Input: dimensioned drawing with shaded views. Units: mm. Origin: part minimum x, y, z. Coordinates: 2 decimals unless noted, no trailing zeros. Write each loop counter-clockwise with the first axis right and the second up, starting at its lowest first coordinate (ties: lowest second). Pieces come first, ordered by that corner, then holes. Notation, with made-up numbers: M 31.25,-34 L 76.25,-34 A16 ccw 76.25,-10 Z; hole C 22,8 d4. An arc over 180 degrees is marked long. Use one line per item in the form item = value.
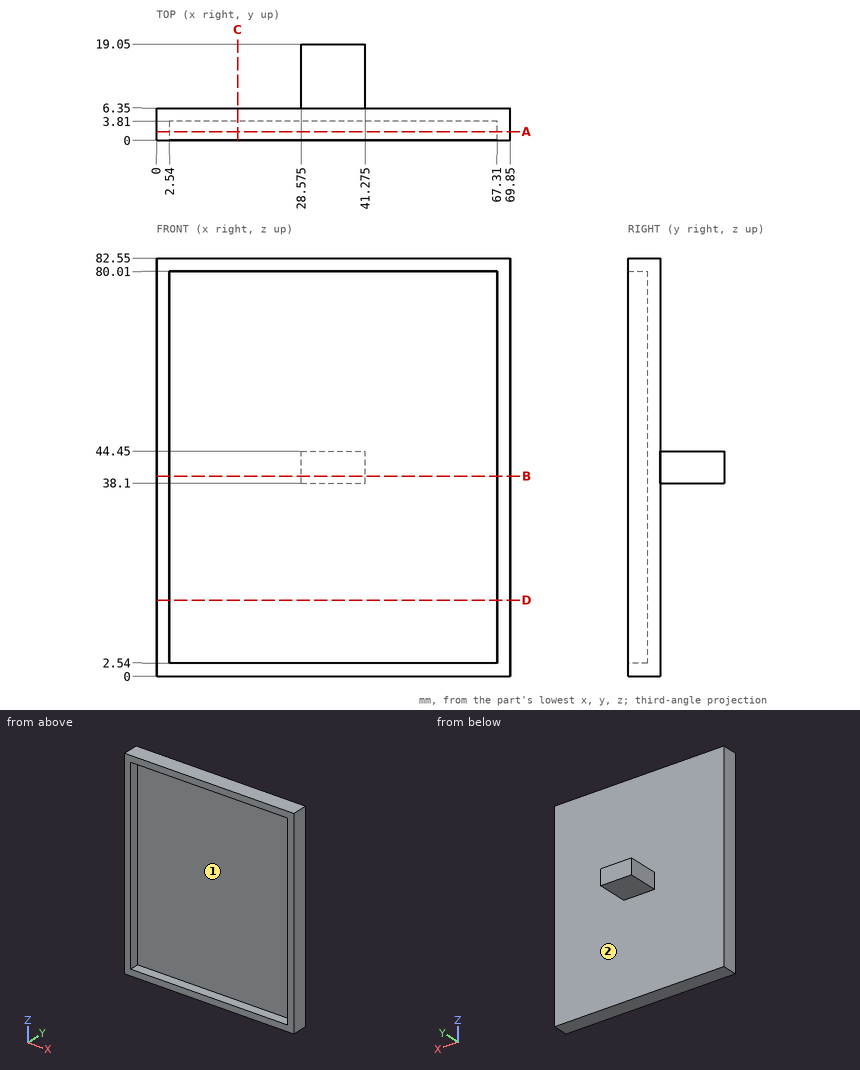
(1) Pull-direction query (X, two-part tool) for the marked faces 1 and 2; classes: pulls with the +X half, pulls with the -X half, needs draft (parallel to the pull), parting line crosses it, or undercut.
Computed:
face_1 = undercut
face_2 = needs draft
(2) Line query: probe 1 along Z at (x, y) = (63, 2); probe 2 along X at (y, z) = (3, 46); probe 3 along Y at (x, z) = (38, 11). Output: solid intervals per line, ascending.
Computed:
probe_1 = 0 to 2.54, 80.01 to 82.55
probe_2 = 0 to 2.54, 67.31 to 69.85
probe_3 = 3.81 to 6.35
(3) First-contact query: pin 1 Ø1 at (x, z) = (9, 21.5) entering from -Y; pin 2 Ø10 at (x, z) = (49, 67.5) entering from +Y; pin 3 Ø5 at (y, z) = (10.5, 42.5) entering from +X (3 decimals). Flat tips, straight axial feed; report the tip coordinate or a pass-through.
Computed:
pin_1 = 3.81
pin_2 = 6.35
pin_3 = 41.275
(4) Section query C-C on x = 16. Return the cut outline in (y, z).
Computed:
outline = M 0,0 L 6.35,0 L 6.35,82.55 L 0,82.55 L 0,80.01 L 3.81,80.01 L 3.81,2.54 L 0,2.54 Z
(5) Section query B-B on z = 39.5. Return the cut outline in (x, y) (3 decimals).
Computed:
outline = M 0,0 L 2.54,0 L 2.54,3.81 L 67.31,3.81 L 67.31,0 L 69.85,0 L 69.85,6.35 L 41.275,6.35 L 41.275,19.05 L 28.575,19.05 L 28.575,6.35 L 0,6.35 Z
(6) Section query D-D on z = 15. Return the cut outline in (x, y).
Computed:
outline = M 0,0 L 2.54,0 L 2.54,3.81 L 67.31,3.81 L 67.31,0 L 69.85,0 L 69.85,6.35 L 0,6.35 Z
(7) Section query A-A on y = 1.75. Return the cut outline in (x, z), plus the area to 3 significant figures.
Computed:
outline = M 0,0 L 69.85,0 L 69.85,82.55 L 0,82.55 Z; hole M 2.54,2.54 L 67.31,2.54 L 67.31,80.01 L 2.54,80.01 Z
area = 748 mm^2
